Source: CAD feature listing. Evaluate the final solid. Frame: model axes, mm. Face numbers are marked on the shaded views. A direction names the side the tool comes from. Give positions to 0.01 mm unless a question says otherwise; leave off trailing zeros. Loops run counter-clockwise (first coordinate to the right, second up) from the corner with the lowest first, then second, coordinate; pieces in that order, holes last. Notation, with made-up numbers: (85, 67) - (139, 67) arc R23 ccw to (139, 103) - close; hole circle Ø9 at (52, 64). An arc over 180 degrees is marked (long way). Put each result on its own line as item: value.
```python
from build123d import *

# Parameters (mm, degrees)
SKETCH1_W           = 0.7
SKETCH1_H           = 20
SKETCH1_W_2         = 1
SKETCH1_W_3         = 8.4
BOSS_EXTRUDE1_DEPTH = 1.5
BOSS_EXTRUDE2_START = 1.5
SKETCH1_3_W         = 1
SKETCH1_3_H         = 20
BOSS_EXTRUDE2_DEPTH = 4


with BuildPart() as part:
    # Sketch1 → Boss-Extrude1 (new body)
    with BuildSketch(Plane(origin=(0, 0, 0), x_dir=(1, 0, 0), z_dir=(0, 1, 0))):
        with Locations((-5.931879195, 2.845637584)):
            Rectangle(SKETCH1_W, SKETCH1_H)
        with Locations((-5.081879195, 2.845637584)):
            Rectangle(SKETCH1_W_2, SKETCH1_H)
        with Locations((-0.381879195, 2.845637584)):
            Rectangle(SKETCH1_W_3, SKETCH1_H)
        with Locations((4.318120805, 2.845637584)):
            Rectangle(SKETCH1_W_2, SKETCH1_H)
        with Locations((5.168120805, 2.845637584)):
            Rectangle(SKETCH1_W, SKETCH1_H)
    extrude(amount=BOSS_EXTRUDE1_DEPTH)

    # Sketch1<3> → Boss-Extrude2 (add)
    with BuildSketch(Plane(origin=(0, 0, 0), x_dir=(1, 0, 0), z_dir=(0, 1, 0)).offset(BOSS_EXTRUDE2_START)):
        with Locations((-5.081879195, 2.845637584)):
            Rectangle(SKETCH1_3_W, SKETCH1_3_H)
        with Locations((4.318120805, 2.845637584)):
            Rectangle(SKETCH1_3_W, SKETCH1_3_H)
    extrude(amount=BOSS_EXTRUDE2_DEPTH)


solid = part.part
```
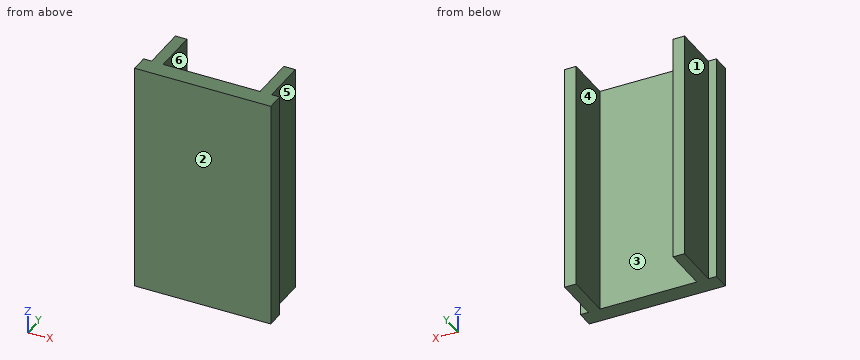
1) Mould query, pull axis X, two halves, no side actions, for the marked faces 1, 2, 3 and 4. Classes: pulls with the +X half, pulls with the -X half, needs draft (parallel to the pull), parting line crosses it, or undercut.
Check result:
face 1: pulls with the -X half
face 2: needs draft
face 3: undercut
face 4: undercut
2) Section query B-B, the plane z = -5.25. Output: boundary loops of the cut face in (x, y), plus the area to 3 significant figures.
Check result:
outline: (-6.28, 0) - (5.52, 0) - (5.52, 1.5) - (4.82, 1.5) - (4.82, 5.5) - (3.82, 5.5) - (3.82, 1.5) - (-4.58, 1.5) - (-4.58, 5.5) - (-5.58, 5.5) - (-5.58, 1.5) - (-6.28, 1.5) - close
area: 25.7 mm²
3) Section query C-C, the plane x = 1.5. Output: boundary loops of the cut face in (y, z), plus the area to 3 significant figures.
Check result:
outline: (0, -12.85) - (1.5, -12.85) - (1.5, 7.15) - (0, 7.15) - close
area: 30.0 mm²
4) Pin query (flat end, axial travel): P1, Ø2, axis at y = 3.5, z = -6, coming from the +X side; P2, Ø1, axis at x = 3, z = -5.5, coming from the +Y side; P3, Ø2, axis at y = 3, z = 1.5, coming from the -X side. Return the tip coordinate at first contact, or that it passes through.
Check result:
P1: x = 4.82
P2: y = 1.5
P3: x = -5.58
5) Access query for the marked faces 5 and 6. Directions: +Z, -Z, +X, -X, +Y, -Y. A direction counts if a zero-diameter tool reaches every point of the face in a straight line with its end or side. Return the directions, or none.
Check result:
face 5: +Z, -Z, +X, +Y
face 6: +Z, -Z, +Y
6) Material intervals for line 1 along X through (y, z) = (4.35, -7); line 2 along Y through (x, z) = (-3.25, 2), sorted ascending. Write a range as [from, to].
Check result:
line 1: [-5.58, -4.58], [3.82, 4.82]
line 2: [0, 1.5]
7) Section query A-A, the plane y = 2.5. Output: boundary loops of the cut face in (x, z).
Check result:
outline: (-5.58, -12.85) - (-4.58, -12.85) - (-4.58, 7.15) - (-5.58, 7.15) - close; (3.82, -12.85) - (4.82, -12.85) - (4.82, 7.15) - (3.82, 7.15) - close
